The model under review builds one solid part; all positions refer to its coordinate system, in mm. Round coordinates to 2 decimals unless told otherwise and drop trailing zeros. Write each loop counter-clockwise with the first axis right and the second up, starting at its lowest first coordinate (ties: lowest second). Pieces come first, ordered by that corner, then holes. Notation, with made-up numbers: M 71.5,72 L 111.5,72 A33 cw 111.5,100 Z; hole C -26.5,10 d4. An arc over 180 degrees is marked long. Write item = value, one per line. Start each with the question number.
Item 1: Take a section at B-B, the plane x = -83.5. Give the boundary of the cut face in (y, z), plus the area to 3 significant figures.
Item 2: Take a section at A-A, the plane y = -47.5. Give the boundary of the cut face in (x, z).
Item 3: To check wall thickness, follow line 1 along X through (y, z) = (47, 0.25); line 2 along X through (y, z) = (-84, 2.25); line 3 along X through (y, z) = (50.5, 2.7). State the ranges of each line that lie inside material, in increasing order.
Item 4: Take a section at C-C, the plane z = 3.2. Give the number of separate pieces and of enclosed holes in the cut face, plus the area to 3 significant figures.
Item 5: The part is to be moulded in two halves that separate along X. For faces 1 (the cylindrical face through (165, 116, 2)), 2 (the flat face through (-13, 26, 0)), say which applies: +X half, -X half, draft (parallel to the pull), parting line (faces both ways), or undercut.
Item 6: For pin 1 Ø1.9 at (y, z) = (140, 2.5) entering from -X; pin 2 Ø2 at (x, z) = (-131.5, 3) entering from -Y; pin 3 Ø1.1 at (x, z) = (-159.5, 3) entering from -Y, all flat-tipped, find the tip position at first contact; note any pin that passes through.
from build123d import *

# Parameters (mm, degrees)
SKETCH2_R           = 1.65
SKETCH2_R_2         = 11
SKETCH2_R_3         = 2.25
SKETCH2_W           = 5
SKETCH2_H           = 5
SKETCH2_H_2         = 7
BOSS_EXTRUDE1_DEPTH = 3.8


with BuildPart() as part:
    # Sketch2 → Boss-Extrude1 (new body)
    with BuildSketch(Plane.XY):
        with BuildLine():
            Line((-170.5, -100), (-163, -100))
            Line((-163, -100), (-163, -95))
            Line((-163, -95), (-158, -95))
            Line((-158, -95), (-158, -100))
            Line((-158, -100), (-137.4, -100))
            ThreePointArc((-137.4, -100), (-135.985786438, -99.414213562), (-135.4, -98))
            Line((-135.4, -98), (-135.4, -22))
            ThreePointArc((-135.4, -22), (-134.814213562, -20.585786438), (-133.4, -20))
            Line((-133.4, -20), (133.4, -20))
            ThreePointArc((133.4, -20), (134.814213562, -20.585786438), (135.4, -22))
            Line((135.4, -22), (135.4, -98))
            ThreePointArc((135.4, -98), (135.985786438, -99.414213562), (137.4, -100))
            Line((137.4, -100), (158, -100))
            Line((158, -100), (158, -95))
            Line((158, -95), (163, -95))
            Line((163, -95), (163, -100))
            Line((163, -100), (170.5, -100))
            Line((170.5, -100), (170.5, -92.5))
            Line((170.5, -92.5), (165.5, -92.5))
            Line((165.5, -92.5), (165.5, -87.5))
            Line((165.5, -87.5), (170.5, -87.5))
            Line((170.5, -87.5), (170.5, -17.8042249))
            Line((170.5, -17.8042249), (165.5, -17.8042249))
            Line((165.5, -17.8042249), (165.5, 67.8042249))
            Line((165.5, 67.8042249), (170.5, 67.8042249))
            Line((170.5, 67.8042249), (170.5, 137.5))
            Line((170.5, 137.5), (165.5, 137.5))
            Line((165.5, 137.5), (165.5, 142.5))
            Line((165.5, 142.5), (170.5, 142.5))
            Line((170.5, 142.5), (170.5, 150))
            Line((170.5, 150), (163, 150))
            Line((163, 150), (163, 145))
            Line((163, 145), (158, 145))
            Line((158, 145), (158, 150))
            Line((158, 150), (137.4, 150))
            ThreePointArc((137.4, 150), (135.985786438, 149.414213562), (135.4, 148))
            Line((135.4, 148), (135.4, 70))
            Line((135.4, 70), (-135.4, 70))
            Line((-135.4, 70), (-135.4, 148))
            ThreePointArc((-135.4, 148), (-135.985786438, 149.414213562), (-137.4, 150))
            Line((-137.4, 150), (-158, 150))
            Line((-158, 150), (-158, 145))
            Line((-158, 145), (-163, 145))
            Line((-163, 145), (-163, 150))
            Line((-163, 150), (-170.5, 150))
            Line((-170.5, 150), (-170.5, 142.5))
            Line((-170.5, 142.5), (-165.5, 142.5))
            Line((-165.5, 142.5), (-165.5, 137.5))
            Line((-165.5, 137.5), (-170.5, 137.5))
            Line((-170.5, 137.5), (-170.5, 67.8042249))
            Line((-170.5, 67.8042249), (-165.5, 67.8042249))
            Line((-165.5, 67.8042249), (-165.5, -17.8042249))
            Line((-165.5, -17.8042249), (-170.5, -17.8042249))
            Line((-170.5, -17.8042249), (-170.5, -87.5))
            Line((-170.5, -87.5), (-165.5, -87.5))
            Line((-165.5, -87.5), (-165.5, -92.5))
            Line((-165.5, -92.5), (-170.5, -92.5))
            Line((-170.5, -92.5), (-170.5, -100))
        make_face()
        with Locations(Location((-168.334802826, 116, 0), (0, 0, 180))):
            Circle(SKETCH2_R, mode=Mode.SUBTRACT)
        with Locations(Location((-139.665197174, 116, 0), (0, 0, 180))):
            Circle(SKETCH2_R, mode=Mode.SUBTRACT)
        with Locations(Location((168.334802826, 116, 0), (0, 0, 180))):
            Circle(SKETCH2_R, mode=Mode.SUBTRACT)
        with Locations(Location((139.665197174, 116, 0), (0, 0, 180))):
            Circle(SKETCH2_R, mode=Mode.SUBTRACT)
        with Locations(Location((154, 116, 0), (0, 0, 180))):
            Circle(SKETCH2_R_2, mode=Mode.SUBTRACT)
        with Locations(Location((-154, 116, 0), (0, 0, 180))):
            Circle(SKETCH2_R_2, mode=Mode.SUBTRACT)
        with Locations(Location((160.5, -0.5, 0), (0, 0, 180))):
            Circle(SKETCH2_R, mode=Mode.SUBTRACT)
        with Locations(Location((160.5, 50.5, 0), (0, 0, 180))):
            Circle(SKETCH2_R, mode=Mode.SUBTRACT)
        with Locations(Location((-160.5, -0.5, 0), (0, 0, 180))):
            Circle(SKETCH2_R, mode=Mode.SUBTRACT)
        with Locations(Location((-160.5, 50.5, 0), (0, 0, 180))):
            Circle(SKETCH2_R, mode=Mode.SUBTRACT)
        with Locations(Location((-35, 10.055, 0), (0, 0, 180))):
            Circle(SKETCH2_R_3, mode=Mode.SUBTRACT)
        with Locations(Location((-35, 39.945, 0), (0, 0, 180))):
            Circle(SKETCH2_R_3, mode=Mode.SUBTRACT)
        with Locations(Location((-59.06, 39.945, 0), (0, 0, 180))):
            Circle(SKETCH2_R_3, mode=Mode.SUBTRACT)
        with Locations(Location((-59.06, 10.055, 0), (0, 0, 180))):
            Circle(SKETCH2_R_3, mode=Mode.SUBTRACT)
        with Locations(Location((59.06, 10.055, 0), (0, 0, 180))):
            Circle(SKETCH2_R_3, mode=Mode.SUBTRACT)
        with Locations(Location((35, 10.055, 0), (0, 0, 180))):
            Circle(SKETCH2_R_3, mode=Mode.SUBTRACT)
        with Locations(Location((35, 39.945, 0), (0, 0, 180))):
            Circle(SKETCH2_R_3, mode=Mode.SUBTRACT)
        with Locations(Location((59.06, 39.945, 0), (0, 0, 180))):
            Circle(SKETCH2_R_3, mode=Mode.SUBTRACT)
        with Locations(Location((168.334802826, -66, 0), (0, 0, 180))):
            Circle(SKETCH2_R, mode=Mode.SUBTRACT)
        with Locations(Location((139.665197174, -66, 0), (0, 0, 180))):
            Circle(SKETCH2_R, mode=Mode.SUBTRACT)
        with Locations(Location((154, -66, 0), (0, 0, 180))):
            Circle(SKETCH2_R_2, mode=Mode.SUBTRACT)
        with Locations(Location((-154, -66, 0), (0, 0, 180))):
            Circle(SKETCH2_R_2, mode=Mode.SUBTRACT)
        with Locations(Location((-139.665197174, -66, 0), (0, 0, 180))):
            Circle(SKETCH2_R, mode=Mode.SUBTRACT)
        with Locations(Location((-168.334802826, -66, 0), (0, 0, 180))):
            Circle(SKETCH2_R, mode=Mode.SUBTRACT)
        with BuildLine():
            Line((-72.45742566, 62.171403079), (-118.05517368, 62.171403079))
            ThreePointArc((-118.05517368, 62.171403079), (-120.883600805, 60.999830204), (-122.05517368, 58.171403079))
            Line((-122.05517368, 58.171403079), (-122.05517368, -8.171403079))
            ThreePointArc((-122.05517368, -8.171403079), (-120.883600805, -10.999830204), (-118.05517368, -12.171403079))
            Line((-118.05517368, -12.171403079), (-72.45742566, -12.171403079))
            ThreePointArc((-72.45742566, -12.171403079), (-69.628998535, -10.999830204), (-68.45742566, -8.171403079))
            Line((-68.45742566, -8.171403079), (-68.45742566, 58.171403079))
            ThreePointArc((-68.45742566, 58.171403079), (-69.628998535, 60.999830204), (-72.45742566, 62.171403079))
        make_face(mode=Mode.SUBTRACT)
        with BuildLine():
            Line((72.45742566, 62.171403079), (118.05517368, 62.171403079))
            ThreePointArc((118.05517368, 62.171403079), (120.883600805, 60.999830204), (122.05517368, 58.171403079))
            Line((122.05517368, 58.171403079), (122.05517368, -8.171403079))
            ThreePointArc((122.05517368, -8.171403079), (120.883600805, -10.999830204), (118.05517368, -12.171403079))
            Line((118.05517368, -12.171403079), (72.45742566, -12.171403079))
            ThreePointArc((72.45742566, -12.171403079), (69.628998535, -10.999830204), (68.45742566, -8.171403079))
            Line((68.45742566, -8.171403079), (68.45742566, 58.171403079))
            ThreePointArc((68.45742566, 58.171403079), (69.628998535, 60.999830204), (72.45742566, 62.171403079))
        make_face(mode=Mode.SUBTRACT)
        with Locations((0, 17.5)):
            Rectangle(SKETCH2_W, SKETCH2_H, mode=Mode.SUBTRACT)
        with Locations((-7.5, 25)):
            Rectangle(SKETCH2_W, SKETCH2_H, mode=Mode.SUBTRACT)
        with Locations((0, 32.5)):
            Rectangle(SKETCH2_W, SKETCH2_H, mode=Mode.SUBTRACT)
        with Locations((7.5, 25)):
            Rectangle(SKETCH2_W, SKETCH2_H, mode=Mode.SUBTRACT)
        with Locations((153, -90)):
            Rectangle(SKETCH2_W, SKETCH2_H, mode=Mode.SUBTRACT)
        with Locations((160.5, -82.5)):
            Rectangle(SKETCH2_W, SKETCH2_H, mode=Mode.SUBTRACT)
        with Locations((-153, -90)):
            Rectangle(SKETCH2_W, SKETCH2_H, mode=Mode.SUBTRACT)
        with Locations((-160.5, -82.5)):
            Rectangle(SKETCH2_W, SKETCH2_H, mode=Mode.SUBTRACT)
        with Locations((160.5, 132.5)):
            Rectangle(SKETCH2_W, SKETCH2_H, mode=Mode.SUBTRACT)
        with Locations((153, 140)):
            Rectangle(SKETCH2_W, SKETCH2_H, mode=Mode.SUBTRACT)
        with Locations((-160.5, 132.5)):
            Rectangle(SKETCH2_W, SKETCH2_H, mode=Mode.SUBTRACT)
        with Locations((-153, 140)):
            Rectangle(SKETCH2_W, SKETCH2_H, mode=Mode.SUBTRACT)
        with Locations((-166, -24.9)):
            Rectangle(SKETCH2_W, SKETCH2_H_2, mode=Mode.SUBTRACT)
        with Locations((-166, -37.9)):
            Rectangle(SKETCH2_W, SKETCH2_H_2, mode=Mode.SUBTRACT)
        with Locations((166, -24.9)):
            Rectangle(SKETCH2_W, SKETCH2_H_2, mode=Mode.SUBTRACT)
        with Locations((166, -37.9)):
            Rectangle(SKETCH2_W, SKETCH2_H_2, mode=Mode.SUBTRACT)
    extrude(amount=BOSS_EXTRUDE1_DEPTH)


solid = part.part
Response values:
q1.outline = M -20,0 L -12.17,0 L -12.17,3.8 L -20,3.8 Z; M 62.17,0 L 70,0 L 70,3.8 L 62.17,3.8 Z
q1.area = 59.5 mm2
q2.outline = M -170.5,0 L -135.4,0 L -135.4,3.8 L -170.5,3.8 Z; M 135.4,0 L 170.5,0 L 170.5,3.8 L 135.4,3.8 Z
q3.line_1 = -165.5 to -122.06, -68.46 to 68.46, 122.06 to 165.5
q3.line_2 = -170.5 to -163, -158 to -135.4, 135.4 to 158, 163 to 170.5
q3.line_3 = -165.5 to -162.15, -158.85 to -122.06, -68.46 to 68.46, 122.06 to 158.85, 162.15 to 165.5
q4.separate_pieces = 1
q4.enclosed_holes = 42
q4.area = 30,700 mm2
q5.face_1 = undercut
q5.face_2 = draft
q6.pin_1 = -165.5
q6.pin_2 = -20
q6.pin_3 = -95
